```python
from build123d import *

# Parameters (mm, degrees)
BLANKSKE_W               = 44
BLANKSKE_H               = 16.7
BLANK_DEPTH              = 4
TOOTHCUTSIM_DEPTH        = 48.232298271
TEETHCUTS_COUNT          = 21
TEETHCUTS_PITCH          = 2.199114855
CROQUIS2_W               = 44
CROQUIS2_H               = 4
CORTAR_EXTRUIR2_DEPTH    = 0.6
CROQUIS3_W               = 2.5
CROQUIS3_H               = 7.1
CORTAR_EXTRUIR3_DEPTH    = 37
CROQUIS4_W               = 5.711786687
CROQUIS4_H               = 1.575
SALIENTE_EXTRUIR4_DEPTH  = 4
CROQUIS5_W               = 1.12
CROQUIS5_H               = 4.3
SALIENTE_EXTRUIR5_DEPTH  = 4.2
CROQUIS14_R              = 1.5
SALIENTE_EXTRUIR11_DEPTH = 2.5
CROQUIS15_W              = 3.088906297
CROQUIS15_H              = 16.1
SALIENTE_EXTRUIR12_DEPTH = 5
CROQUIS16_W              = 2.855893344
CROQUIS16_H              = 16.1
SALIENTE_EXTRUIR13_DEPTH = 5
SALIENTE_EXTRUIR14_DEPTH = 2
CROQUIS18_W              = 4.2
CROQUIS18_H              = 4.3
SALIENTE_EXTRUIR15_DEPTH = 2
CROQUIS19_W              = 2.855893344
CROQUIS19_H              = 14
SALIENTE_EXTRUIR16_DEPTH = 8
CROQUIS20_W              = 2.855893344
CROQUIS20_H              = 24.1
SALIENTE_EXTRUIR18_DEPTH = 2
SALIENTE_EXTRUIR19_DEPTH = 3
CROQUIS31_W              = 2.855893344
CROQUIS31_H              = 27.1
SALIENTE_EXTRUIR20_DEPTH = 16
CROQUIS32_W              = 3.088906297
CROQUIS32_H              = 27.1
SALIENTE_EXTRUIR21_DEPTH = 16
REDONDEO3_R              = 3
REDONDEO4_R              = 3.1


# Some blends are built 0.0001 mm under size
with BuildPart() as part:
    # BlankSke → Blank (new body)
    with BuildSketch(Plane.XY):
        with Locations((22, 8.35)):
            Rectangle(BLANKSKE_W, BLANKSKE_H)
    extrude(amount=-BLANK_DEPTH)

    # TooCutSkeSim → ToothCutSim (cut, through all)
    with BuildSketch(Plane.XY):
        Polygon((0.312304759, 15.125), (-0.312304759, 15.125), (-0.894802722, 16.7254), (0.894802722, 16.7254), align=None)
    toothcutsim = extrude(amount=-TOOTHCUTSIM_DEPTH, mode=Mode.SUBTRACT)

    # TeethCuts: ToothCutSim ×21
    with Locations(*[(i * TEETHCUTS_PITCH, 0, 0) for i in range(1, TEETHCUTS_COUNT)]):
        add(toothcutsim, mode=Mode.SUBTRACT)

    # Croquis2 → Cortar-Extruir2 (cut)
    with BuildSketch(Plane.XZ):
        with Locations((22, -2)):
            Rectangle(CROQUIS2_W, CROQUIS2_H)
    extrude(amount=-CORTAR_EXTRUIR2_DEPTH, mode=Mode.SUBTRACT)

    # Croquis3 → Cortar-Extruir3 (cut)
    with BuildSketch(Plane(origin=(44, 0, 0), x_dir=(0, 0, -1), z_dir=(1, 0, 0))):
        with Locations((2.75, 7.8625)):
            Rectangle(CROQUIS3_W, CROQUIS3_H)
    extrude(amount=-CORTAR_EXTRUIR3_DEPTH, mode=Mode.SUBTRACT)

    # Croquis4 → Saliente-Extruir4 (add)
    with BuildSketch(Plane.XY):
        with Locations((2.855893344, 15.9125)):
            Rectangle(CROQUIS4_W, CROQUIS4_H)
    extrude(amount=-SALIENTE_EXTRUIR4_DEPTH)

    # Croquis5 → Saliente-Extruir5 (add)
    with BuildSketch(Plane(origin=(0, 0, -1.5), x_dir=(-1, 0, 0), z_dir=(0, 0, -1))):
        with Locations((-39.01, 7.8625)):
            Rectangle(CROQUIS5_W, CROQUIS5_H)
    extrude(amount=SALIENTE_EXTRUIR5_DEPTH)

    # Croquis14 → Saliente-Extruir11 (add)
    with BuildSketch(Plane(origin=(39.57, 0, 0), x_dir=(0, 0, -1), z_dir=(1, 0, 0))):
        with Locations(Location((3.6, 7.8625, 0), (0, 0, 180))):
            Circle(CROQUIS14_R)
    extrude(amount=SALIENTE_EXTRUIR11_DEPTH)

    # Croquis15 → Saliente-Extruir12 (add)
    with BuildSketch(Plane.XY):
        with Locations((1.544453149, 8.65)):
            Rectangle(CROQUIS15_W, CROQUIS15_H)
    extrude(amount=SALIENTE_EXTRUIR12_DEPTH)

    # Croquis16 → Saliente-Extruir13 (add)
    with BuildSketch(Plane(origin=(0, 0, -4), x_dir=(-1, 0, 0), z_dir=(0, 0, -1))):
        with Locations((-1.427946672, 8.65)):
            Rectangle(CROQUIS16_W, CROQUIS16_H)
    extrude(amount=SALIENTE_EXTRUIR13_DEPTH)

    # Croquis17 → Saliente-Extruir14 (add)
    with BuildSketch(Plane(origin=(0, 0, -4), x_dir=(-1, 0, 0), z_dir=(0, 0, -1))):
        Polygon((-44, 0.6), (-2.855893344, 0.6), (-2.855893344, 16.7), (-5.711786687, 16.7), (-6.285039806, 15.125), (-6.909649324, 15.125), (-7.482902443, 16.7), (-7.910901542, 16.7), (-8.484154661, 15.125), (-9.108764179, 15.125), (-9.682017298, 16.7), (-10.110016397, 16.7), (-10.683269516, 15.125), (-11.307879034, 15.125), (-11.881132153, 16.7), (-12.309131252, 16.7), (-12.882384371, 15.125), (-13.506993889, 15.125), (-14.080247008, 16.7), (-14.508246107, 16.7), (-15.081499226, 15.125), (-15.706108744, 15.125), (-16.279361863, 16.7), (-16.707360962, 16.7), (-17.280614081, 15.125), (-17.905223599, 15.125), (-18.478476718, 16.7), (-18.906475817, 16.7), (-19.479728936, 15.125), (-20.104338454, 15.125), (-20.677591573, 16.7), (-21.105590672, 16.7), (-21.678843791, 15.125), (-22.303453309, 15.125), (-22.876706428, 16.7), (-23.304705527, 16.7), (-23.877958646, 15.125), (-24.502568164, 15.125), (-25.075821283, 16.7), (-25.503820382, 16.7), (-26.077073501, 15.125), (-26.701683019, 15.125), (-27.274936138, 16.7), (-27.702935237, 16.7), (-28.276188356, 15.125), (-28.900797874, 15.125), (-29.474050993, 16.7), (-29.902050092, 16.7), (-30.475303211, 15.125), (-31.099912729, 15.125), (-31.673165848, 16.7), (-32.101164947, 16.7), (-32.674418066, 15.125), (-33.299027584, 15.125), (-33.872280703, 16.7), (-34.300279802, 16.7), (-34.873532921, 15.125), (-35.498142439, 15.125), (-36.071395558, 16.7), (-36.499394657, 16.7), (-37.072647776, 15.125), (-37.697257294, 15.125), (-38.270510413, 16.7), (-38.698509512, 16.7), (-39.271762631, 15.125), (-39.896372149, 15.125), (-40.469625268, 16.7), (-40.897624367, 16.7), (-41.470877486, 15.125), (-42.095487004, 15.125), (-42.668740123, 16.7), (-43.096739222, 16.7), (-43.669992341, 15.125), (-44, 15.125), (-44, 11.4125), (-7, 11.4125), (-7, 4.3125), (-44, 4.3125), align=None)
    extrude(amount=SALIENTE_EXTRUIR14_DEPTH)

    # Croquis18 → Saliente-Extruir15 (add)
    with BuildSketch(Plane.ZY.offset(-38.45)):
        with Locations((-3.6, 7.8625)):
            Rectangle(CROQUIS18_W, CROQUIS18_H)
    extrude(amount=SALIENTE_EXTRUIR15_DEPTH)

    # Croquis19 → Saliente-Extruir16 (add)
    with BuildSketch(Plane(origin=(0, 16.7, 0), x_dir=(1, 0, 0), z_dir=(0, 1, 0))):
        with Locations((1.427946672, 2)):
            Rectangle(CROQUIS19_W, CROQUIS19_H)
    extrude(amount=SALIENTE_EXTRUIR16_DEPTH)

    # Croquis20 → Saliente-Extruir18 (add)
    with BuildSketch(Plane(origin=(0, 0, -9), x_dir=(-1, 0, 0), z_dir=(0, 0, -1))):
        with Locations((-1.427946672, 12.65)):
            Rectangle(CROQUIS20_W, CROQUIS20_H)
    extrude(amount=SALIENTE_EXTRUIR18_DEPTH)

    # Croquis21 → Saliente-Extruir19 (add)
    with BuildSketch(Plane.XZ.offset(-0.6)):
        Polygon((3.088906297, 0), (2.855893344, -6), (2.855893344, -11), (0, -11), (0, 5), (3.088906297, 5), align=None)
    extrude(amount=SALIENTE_EXTRUIR19_DEPTH)

    # Croquis31 → Saliente-Extruir20 (add)
    with BuildSketch(Plane(origin=(0, 0, -11), x_dir=(-1, 0, 0), z_dir=(0, 0, -1))):
        with Locations((-1.427946672, 11.15)):
            Rectangle(CROQUIS31_W, CROQUIS31_H)
    extrude(amount=-SALIENTE_EXTRUIR20_DEPTH)

    # Croquis32 → Saliente-Extruir21 (add)
    with BuildSketch(Plane.XY.offset(5)):
        with Locations((1.544453149, 11.15)):
            Rectangle(CROQUIS32_W, CROQUIS32_H)
    extrude(amount=-SALIENTE_EXTRUIR21_DEPTH)

    # Redondeo3
    redondeo3_edges = [part.edges().sort_by_distance(p)[0] for p in [
        (23.544453148, 0.6, -6),
        (23.544453148, 0.6, 0),
    ]]
    fillet(redondeo3_edges, radius=REDONDEO3_R - 0.0001)  # a hair under: the kernel refuses the full size

    # Redondeo4
    # the kernel refuses this fillet: 3.1 mm, written as the material it takes off along each edge
    with BuildSketch(Plane(origin=(3.088906297, -2.4, -18.75), x_dir=(0, 1, 0), z_dir=(0, 0, 1))) as redondeo4_piece_1_section:
        with BuildLine():
            CenterArc((REDONDEO4_R, REDONDEO4_R), REDONDEO4_R, 180, 90)
            Line((0, REDONDEO4_R), (0, 0))
            Line((0, 0), (REDONDEO4_R, 0))
        make_face()
    redondeo4_piece_1 = extrude(amount=31.5, mode=Mode.PRIVATE)
    redondeo4_piece_1 = redondeo4_piece_1 - Plane(origin=(2.386115021, 3.5999, -3.0001), x_dir=(0, -1, 0), z_dir=(-1, 0, 0)) * Cylinder(2.9999, 76, mode=Mode.PRIVATE)
    add(redondeo4_piece_1, mode=Mode.SUBTRACT)
    with BuildSketch(Plane(origin=(3.088906297, -10.15, 5), x_dir=(0, 0, -1), z_dir=(0, 1, 0)), Plane(origin=(3.088906297, 32.45, -11), x_dir=(0, 0, 1), z_dir=(0, -1, 0))) as redondeo4_piece_2:
        with BuildLine():
            CenterArc((REDONDEO4_R, REDONDEO4_R), REDONDEO4_R, 180, 90)
            Line((0, REDONDEO4_R), (0, 0))
            Line((0, 0), (REDONDEO4_R, 0))
        make_face()
    extrude(amount=42.6, mode=Mode.SUBTRACT)
    with BuildSketch(Plane(origin=(3.088906297, 24.7, 12.75), x_dir=(0, -1, 0), z_dir=(0, 0, -1))) as redondeo4_piece_3:
        with BuildLine():
            CenterArc((REDONDEO4_R, REDONDEO4_R), REDONDEO4_R, 180, 90)
            Line((0, REDONDEO4_R), (0, 0))
            Line((0, 0), (REDONDEO4_R, 0))
        make_face()
    extrude(amount=31.5, mode=Mode.SUBTRACT)


solid = part.part
```
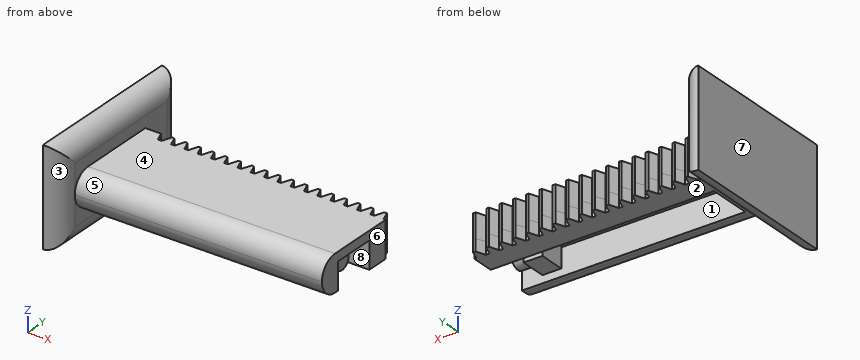
Verification items for the finished model (mm, model axes). Face numbers are marked on the shaded views. A direction names the side the tool comes from. Coordinates: 2 decimals unless noted, no trailing zeros. Write each loop counter-clockwise with the first axis right and the second up, starting at its lowest first coordinate (ties: lowest second). Pieces come first, ordered by that corner, then holes. Notation, with made-up numbers: M 15,50.25 L 22,50.25 A12 ccw 22,57.25 Z; hole C 47.25,86 d9. An arc over 180 degrees is marked long. Answer as a JSON object with one key per item and string values. Group by question number.
(1) Gauge pin test, flat ends, axial feed: pin 1 (1.3 mm diameter, centred on y = 6, z = -3, fed in from +X); pin 2 (5 mm diameter, centred on x = 21.5, z = 1.5, fed in from +Y); pin 3 (5 mm diameter, centred on x = 23.5, z = -3, fed in from -Y). Record the tip position at first contact, or that the pin passes through.
(2) Cross-section at A-A, the plane y = 3. Record the cut outline in (x, z), and give its area (3 significant figures).
(3) Material ranges on line 1 (Z direction, x = 15.5, y = 9); line 2 (Z direction, x = 41.5, y = 3.75); line 3 (X direction, y = 13.25, z = 0.5), recorded low to high.
(4) Tool access check on the marked faces 4, 5, 6, 7 and 8. Record the directions out of +Z, -Z, +X, -X, +Y, -Y that give a thin tool (end or side, any length) a straight path to the whole face; none if there is none.
(5) Release check for a two-part mould opening along Y. For the marked faces 1, 2 and 3 record: +Y half, -Y half, draft (parallel to the pull), parting line (faces both ways), or undercut.
(6) Cross-section at B-B, the plane z = -10. Record the cut outline in (x, y).
Reply:
{
 "1": {"pin 1": "x = 42.07", "pin 2": "y = 16.7", "pin 3": "y = 0.6"},
 "2": {"outline": "M 0,-11 A3.1 ccw 3.09,-7.9 L 3.09,-5.94 L 44,-5.94 L 44,-0.06 L 3.09,-0.06 L 3.09,1.9 A3.1 ccw 0,5 Z", "area": "286 mm²"},
 "3": {"line 1": "-1.5 to 0", "line 2": "-6 to 0", "line 3": "0 to 3.09"},
 "4": {"face 4": "+Z, +X, +Y, -Y", "face 5": "+Z, +X, -Y", "face 6": "+Z, -Z, +X, +Y, -Y", "face 7": "+Z, -Z, -X, +Y, -Y", "face 8": "-Z, +X"},
 "5": {"face 1": "undercut", "face 2": "draft", "face 3": "-Y half"},
 "6": {"outline": "M 0,-2.4 A3.1 ccw 2.27,-1.4 L 2.27,23.7 A3.1 ccw 0,24.7 Z"}
}
